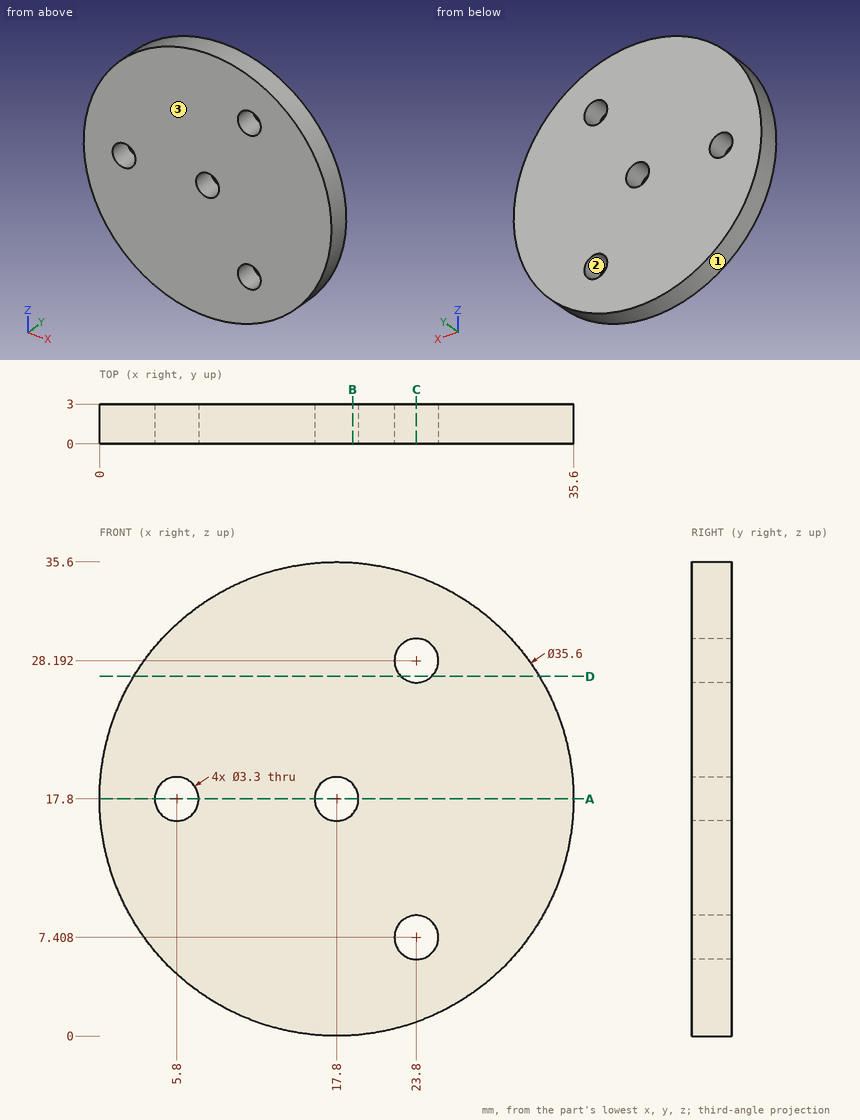
Here's the drawing with two shaded views (mm, measured from the low corner). I have some questions. Coordinates: 2 decimals unless noted, no trailing zeros. Write each loop counter-clockwise with the first axis right and the second up, starting at its lowest first coordinate (ties: lowest second). Pieces come first, ordered by that corner, then holes. Notation, with made-up numbers: (-11, 79.5) -> (18, 79.5) arc R31 cw to (18, 107.5) -> close; hole circle Ø3 at (7.5, 30). An arc over 180 degrees is marked (long way). Write item = value, one per line. Start each with the question number.
(1) I want a section at A-A (z = 17.8). Please give me the cut outline in (x, y), plus the area to 3 significant figures.
(2) I want a section at C-C (x = 23.8). Please give me the cut outline in (y, z).
(3) I want a section at B-B (x = 19). Please give me the cut outline in (y, z).
(4) I want a section at D-D (z = 27). Please give me the cut outline in (x, y).
(5) Will these pins go through, and if not, where does the flat tip stop? pin 1 (1.5 mm diameter, centred on x = 16, y = 1.5, fed in from -Z); pin 2 (3 mm diameter, centred on x = 5.8, z = 17.8, fed in from +Y).
(6) We'd pull the mould along Z, two halves only. Please class the marked faces 1, 2 and 3: released by +Z, released by -Z, zero draft, split by the parting line, or undercut.
(7) I need wall thicknesses on line 1 (X direction, y = 0.55, z = 19); line 2 (Z direction, x = 23.8, y = 2.05); line 3 (X direction, y = 1.2, z = 18). Which ranges of each line are inside material? Lowest first, please. Write a range as [from, to].
Result set:
q1.outline = (0, 0) -> (4.15, 0) -> (4.15, 3) -> (0, 3) -> close; (7.45, 0) -> (16.15, 0) -> (16.15, 3) -> (7.45, 3) -> close; (19.45, 0) -> (35.6, 0) -> (35.6, 3) -> (19.45, 3) -> close
q1.area = 87.0 mm2
q2.outline = (0, 1.04) -> (3, 1.04) -> (3, 5.76) -> (0, 5.76) -> close; (0, 9.06) -> (3, 9.06) -> (3, 26.54) -> (0, 26.54) -> close; (0, 29.84) -> (3, 29.84) -> (3, 34.56) -> (0, 34.56) -> close
q3.outline = (0, 0.04) -> (3, 0.04) -> (3, 16.67) -> (0, 16.67) -> close; (0, 18.93) -> (3, 18.93) -> (3, 35.56) -> (0, 35.56) -> close
q4.outline = (2.56, 0) -> (22.66, 0) -> (22.66, 3) -> (2.56, 3) -> close; (24.94, 0) -> (33.04, 0) -> (33.04, 3) -> (24.94, 3) -> close
q5.pin_1 = 0.03
q5.pin_2 = through
q6.face_1 = split by the parting line
q6.face_2 = undercut
q6.face_3 = zero draft
q7.line_1 = [0.04, 4.67], [6.93, 16.67], [18.93, 35.56]
q7.line_2 = [1.04, 5.76], [9.06, 26.54], [29.84, 34.56]
q7.line_3 = [0, 4.16], [7.44, 16.16], [19.44, 35.6]
